Can you work these out from the model? Positions are in its coordinate system, mm. A direction names the side the tool comes from. Round coordinates to 2 decimals unless told otherwise and drop trailing zeros. Write each loop counter-clockwise with the first axis right and the second up, starting at its lowest first coordinate (ties: lowest second). Pieces come first, ordered by that corner, then holes. Notation, with made-up numbers: M -17.5,6 L 22.5,6 A17 ccw 22.5,38 Z; hole C 35.5,-12 d2. An arc over 180 degrees is marked long. Answer as a JSON object with one key per item and string values. Group by question number.
1) I'm going to push flat-ended pins straight in: pin 1 Ø12.5 at (x, y) = (38.5, 18) entering from +Z; pin 2 Ø11 at (x, y) = (8.5, 8.5) entering from +Z; pin 3 Ø1.6 at (x, z) = (9, 34.5) entering from -Y (3 decimals); pin 4 Ø1.2 at (y, z) = (14, 34.5) entering from -X. Where does each tip first touch, or does it pass through?
2) Suppose I cut it at B-B, the plane y = 17.75. Write out the boundary of the cut face in (x, z).
3) Suppose I cut it at A-A, the plane x = 35.23. Write out the boundary of the cut face in (y, z) (3 decimals), and give its area (3 significant figures).
4) Suppose I cut it at C-C, the plane x = 11.5. Write out the boundary of the cut face in (y, z) (3 decimals), and give its area (3 significant figures).
5) Please list where these lines run through material, in increasing order: L1, parallel to Z at x = 37.5, y = 19.25; L2, parallel to Z at x = 6.5, y = 2.5; L3, parallel to X at y = 6.5, z = 1.5. Write a range as [from, to].
6) Suppose I cut it at D-D, the plane y = 7.75. Write out the boundary of the cut face in (x, z).
7) On a 3-axis mill with a long thin cutter (end or side, diameter ignored), from which of +Z, -Z, +X, -X, +Y, -Y can I reach the whole of each face in a straight line? I mean faces 1 (the flat face through (10, 21.365, 34)), 2 (the flat face through (11, 3, 1.5)), 3 (the flat face through (11, 12, 0)). Say none if no direction works.
from build123d import *

# Parameters (mm, degrees)
SKETCH_1_W           = 45.23
SKETCH_1_H           = 24.73
EXTRUDE_1_DEPTH      = 35
CUT_EXTRUDE_1_DEPTH  = 3
SKETCH_5_W           = 1.897849624
SKETCH_5_H           = 24.73
CUT_EXTRUDE_3_DEPTH  = 3
EXTRUDE_2_DEPTH      = 17.9
EXTRUDE_2_DEPTH_BACK = 18.6
EXTRUDE_2_START      = 17.5
SKETCH_3_R           = 3
SKETCH_4_W           = 30.897849624
SKETCH_4_H           = 5
CUT_EXTRUDE_2_DEPTH  = 1.5
CHAMFER_1_SIZE       = 2.5
FILLET_1_R           = 2
SKETCH_6_W           = 10
SKETCH_6_H           = 18
CUT_EXTRUDE_4_DEPTH  = 1.5
CHAMFER_2_SIZE       = 0.5


with BuildPart() as part:
    # 草图1 → 凸台-拉伸1 (new body)
    with BuildSketch(Plane.XY):
        with Locations((22.615, 12.365)):
            Rectangle(SKETCH_1_W, SKETCH_1_H)
    extrude(amount=EXTRUDE_1_DEPTH)

    # 草图2 → 切除-拉伸1 (cut)
    with BuildSketch(Plane.XY):
        with BuildLine():
            Line((45.23, 24.73), (30.897849624, 24.73))
            ThreePointArc((30.897849624, 24.73), (20.23, 12.365), (30.897849624, 0))
            Line((30.897849624, 0), (45.23, 0))
            Line((45.23, 0), (45.23, 24.73))
        make_face()
    cut_extrude_1 = extrude(amount=CUT_EXTRUDE_1_DEPTH, mode=Mode.SUBTRACT)

    # 草图5 → 切除-拉伸3 (cut)
    with BuildSketch(Plane.XY):
        with Locations((29.948924812, 12.365)):
            Rectangle(SKETCH_5_W, SKETCH_5_H)
    cut_extrude_3 = extrude(amount=CUT_EXTRUDE_3_DEPTH, mode=Mode.SUBTRACT)

    # 镜向1: 切除-拉伸1, 切除-拉伸3 across plane
    add(cut_extrude_1.mirror(Plane.XY.offset(17.5)), mode=Mode.SUBTRACT)
    add(cut_extrude_3.mirror(Plane.XY.offset(17.5)), mode=Mode.SUBTRACT)

    # 草图3 → 凸台-拉伸2 (add, two sides: drawn at the far end of the back side and taken through both)
    with BuildSketch(Plane.XY.offset(EXTRUDE_2_START - EXTRUDE_2_DEPTH_BACK)):
        with Locations((35.23, 12.365)):
            Circle(SKETCH_3_R)
    extrude(amount=EXTRUDE_2_DEPTH + EXTRUDE_2_DEPTH_BACK)

    # 草图4 → 切除-拉伸2 (cut)
    with BuildSketch(Plane.XY):
        with Locations((15.448924812, 22.23)):
            Rectangle(SKETCH_4_W, SKETCH_4_H)
        with Locations((15.448924812, 2.5)):
            Rectangle(SKETCH_4_W, SKETCH_4_H)
    extrude(amount=CUT_EXTRUDE_2_DEPTH, mode=Mode.SUBTRACT)

    # 倒角1
    chamfer_1_edges = [part.edges().sort_by_distance(p)[0] for p in [
        (45.23, 0, 17.5),
        (45.23, 24.73, 17.5),
    ]]
    chamfer(chamfer_1_edges, length=CHAMFER_1_SIZE)

    # 圆角1
    fillet_1_edges = [part.edges().sort_by_distance(p)[0] for p in [
        (0, 24.73, 18.25),
        (0, 0, 18.25),
    ]]
    fillet(fillet_1_edges, radius=FILLET_1_R)

    # 草图6 → 切除-拉伸4 (cut)
    with BuildSketch(Plane.XY.offset(35)):
        with BuildLine():
            Line((29, 24.73), (2, 24.73))
            ThreePointArc((2, 24.73), (0.585786438, 24.144213562), (0, 22.73))
            Line((0, 22.73), (0, 2))
            ThreePointArc((0, 2), (0.585786438, 0.585786438), (2, 0))
            Line((2, 0), (29, 0))
            Line((29, 0), (29, 0.434488695))
            ThreePointArc((29, 0.434488695), (20.23, 12.365), (29, 24.295511305))
            Line((29, 24.295511305), (29, 24.73))
        make_face()
        with Locations((10, 12.365)):
            Rectangle(SKETCH_6_W, SKETCH_6_H, mode=Mode.SUBTRACT)
    extrude(amount=-CUT_EXTRUDE_4_DEPTH, mode=Mode.SUBTRACT)

    # 倒角2
    chamfer_2_edges = [part.edges().sort_by_distance(p)[0] for p in [
        (0, 21.23, 1.5),
        (15.5, 24.73, 1.5),
        (0, 12.365, 0),
        (0, 3.5, 1.5),
        (15.5, 0, 1.5),
        (15.5, 24.73, 33.5),
        (15.5, 0, 33.5),
    ]]
    chamfer(chamfer_2_edges, length=CHAMFER_2_SIZE)


solid = part.part
Results:
{
 "1": {"pin 1": "z = 35.4", "pin 2": "z = 35", "pin 3": "y = 3.365", "pin 4": "x = 5"},
 "2": {"outline": "M 0,0.5 L 0.5,0 L 21.45,0 L 21.45,3 L 45.23,3 L 45.23,32 L 21.45,32 L 21.45,33.5 L 15,33.5 L 15,35 L 5,35 L 5,33.5 L 0.5,33.5 L 0,33 Z"},
 "3": {"outline": "M 0,3 L 9.365,3 L 9.365,-1.1 L 15.365,-1.1 L 15.365,3 L 24.73,3 L 24.73,32 L 15.365,32 L 15.365,35.4 L 9.365,35.4 L 9.365,32 L 0,32 Z", "area": "762 mm^2"},
 "4": {"outline": "M 0,2 L 0.5,1.5 L 5,1.5 L 5,0 L 19.73,0 L 19.73,1.5 L 24.23,1.5 L 24.73,2 L 24.73,33 L 24.23,33.5 L 21.365,33.5 L 21.365,35 L 3.365,35 L 3.365,33.5 L 0.5,33.5 L 0,33 Z", "area": "840 mm^2"},
 "5": {"L1": "[3, 32]", "L2": "[1.5, 33.5]", "L3": "[0, 21.69]"},
 "6": {"outline": "M 0,0.5 L 0.5,0 L 21.11,0 L 21.11,3 L 45.23,3 L 45.23,32 L 21.11,32 L 21.11,33.5 L 15,33.5 L 15,35 L 5,35 L 5,33.5 L 0.5,33.5 L 0,33 Z"},
 "7": {"face 1": "+Z, +X, -X, +Y", "face 2": "-Z, +X, -X, -Y", "face 3": "-Z, -X, +Y, -Y"}
}
